```python
from build123d import *

# Parameters (mm, degrees)
BOSS_EXTRU_1_DEPTH      = 2850
ESQUISSE3_R             = 4
ENL_V_MAT_EXTRU_1_DEPTH = 10


with BuildPart() as part:
    # Esquisse1 → Boss.-Extru.1 (new body)
    with BuildSketch(Plane.XY):
        Polygon((-12, -79.697824129), (23, -79.697824129), (23, -69.697824129), (3, -69.697824129), (58.522190754, -37.642072351), (43.522190754, -37.642072351), (-12, -69.697824129), align=None)
    extrude(amount=BOSS_EXTRU_1_DEPTH)

    # Esquisse3 → Enlèv. mat.-Extru.1 (cut)
    with BuildSketch(Plane.XZ.offset(79.697824129)):
        with Locations(Location((14, 90, 0), (0, 0, 270))):
            Circle(ESQUISSE3_R)
        with Locations(Location((14, 290, 0), (0, 0, 270))):
            Circle(ESQUISSE3_R)
        with Locations(Location((14, 490, 0), (0, 0, 270))):
            Circle(ESQUISSE3_R)
        with Locations(Location((14, 690, 0), (0, 0, 270))):
            Circle(ESQUISSE3_R)
        with Locations(Location((14, 890, 0), (0, 0, 270))):
            Circle(ESQUISSE3_R)
        with Locations(Location((14, 1090, 0), (0, 0, 270))):
            Circle(ESQUISSE3_R)
        with Locations(Location((14, 1290, 0), (0, 0, 270))):
            Circle(ESQUISSE3_R)
        with Locations(Location((14, 1490, 0), (0, 0, 270))):
            Circle(ESQUISSE3_R)
        with Locations(Location((14, 1690, 0), (0, 0, 270))):
            Circle(ESQUISSE3_R)
        with Locations(Location((14, 1890, 0), (0, 0, 270))):
            Circle(ESQUISSE3_R)
        with Locations(Location((14, 2090, 0), (0, 0, 270))):
            Circle(ESQUISSE3_R)
        with Locations(Location((14, 2290, 0), (0, 0, 270))):
            Circle(ESQUISSE3_R)
        with Locations(Location((14, 2490, 0), (0, 0, 270))):
            Circle(ESQUISSE3_R)
        with Locations(Location((14, 2690, 0), (0, 0, 270))):
            Circle(ESQUISSE3_R)
    extrude(amount=-ENL_V_MAT_EXTRU_1_DEPTH, mode=Mode.SUBTRACT)


solid = part.part
```
Check sheet for the modelled part. Datum: model origin and axes. Units: mm. Round coordinates to 2 decimals unless told otherwise and drop trailing zeros. Order: outer loops, then holes, each group sorted by start corner. A loop starts at its lowest first (then second) coordinate and runs counter-clockwise, first axis right, second up. Notation, with made-up numbers: (4.5, 34) - (29.5, 34) arc R29 ccw to (29.5, 73) - close; hole circle Ø9 at (-33, 19). An arc over 180 degrees is marked (long way). Answer as CSV lines item,"result". Start each with the question number.
1) Section check A-A (z = 1748). Record the cut outline in (x, y).
2) Draft check along Y on faces 1 (the face through (30.372, -53.894, 1405.05)), 2 (the face through (16.15, -53.446, 1405.05)). Enter one of: +Y half, -Y half, draft (parallel to the pull), parting line (faces both ways), or undercut.
3) Depth check by flat-ended pin: pin 1 (5 mm diameter, centred on x = 14, z = 90, fed in from +Y); pin 2 (5 mm diameter, centred on x = 14, z = 2090, fed in from -Y); pin 3 (10 mm diameter, centred on x = 12, z = 1160, fed in from +Y); pin 4 (10.5 mm diameter, centred on x = 14, z = 2290, fed in from -Y). Enter the tip coordinate at first touch or a pass-through.
4) Section check B-B (y = -47). Record the cut outline in (x, z).
5) Scan lines: probe 1 along X at (y, z) = (-76.75, 90); probe 2 along X at (y, z) = (-71, 1812.5); probe 3 along Y at (x, z) = (16.5, 370.5). Record each from-to range of solid material in increasing order.
Determined:
1,outline,"(-12, -79.7) - (23, -79.7) - (23, -69.7) - (3, -69.7) - (58.52, -37.64) - (43.52, -37.64) - (-12, -69.7) - close"
2,face 1,"undercut"
2,face 2,"+Y half"
3,pin 1,"y = -53.24"
3,pin 2,"y = -64.79"
3,pin 3,"y = -52.95"
3,pin 4,"y = -79.7"
4,outline,"(27.31, 0) - (42.31, 0) - (42.31, 2850) - (27.31, 2850) - close"
5,probe 1,"-12 to 10, 18 to 23"
5,probe 2,"-12 to 23"
5,probe 3,"-79.7 to -69.7, -61.9 to -53.24"
